Drawing for the job (mm, zero at the part's lowest x, y, z). Round coordinates to 2 decimals unless told otherwise and drop trailing zeros. Write each loop counter-clockwise with the first axis right and the second up, starting at its lowest first coordinate (ties: lowest second). Pieces come first, ordered by that corner, then holes. Notation, with made-up numbers: (21.25, 56.5) - (41.25, 56.5) arc R26 cw to (41.25, 77.5) - close; hole circle Ø7 at (87, 31). An arc over 180 degrees is marked (long way). One line per question, with ' | ' between items.
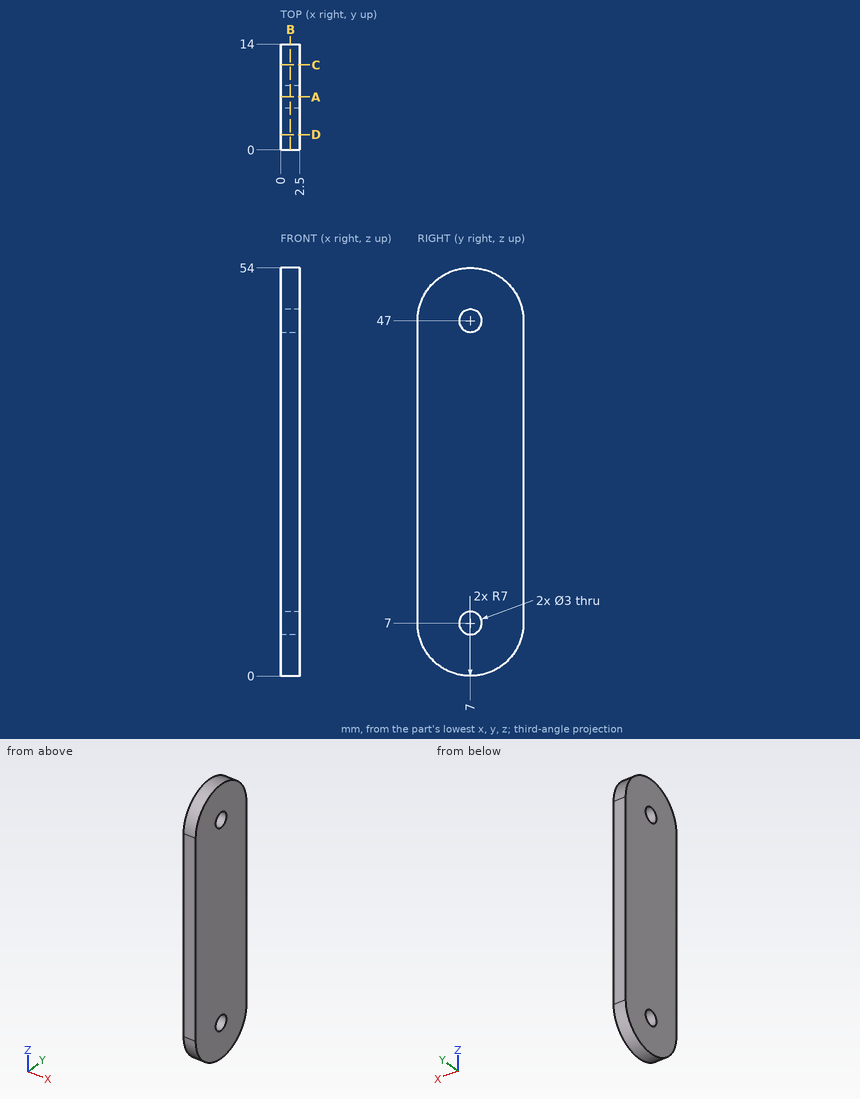
Q1. Saw through at B-B, the plane x = 1.3. List the corners of the cut face in (y, z), then the cut area to 3 significant figures.
Found:
outline: (0, 7) arc R7 ccw to (14, 7) - (14, 47) arc R7 ccw to (0, 47) - close; hole circle Ø3 at (7, 7); hole circle Ø3 at (7, 47) | area: 700 mm^2
Q2. Saw through at A-A, the plane y = 7. List the corners of the cut face in (x, z), then the cut area to 3 significant figures.
Found:
outline: (0, 0) - (2.5, 0) - (2.5, 5.5) - (0, 5.5) - close; (0, 8.5) - (2.5, 8.5) - (2.5, 45.5) - (0, 45.5) - close; (0, 48.5) - (2.5, 48.5) - (2.5, 54) - (0, 54) - close | area: 120 mm^2
Q3. Drill centre lines: L1, parallel to Y at x = 0.75, z = 7; L2, parallel to Z at x = 1.5, y = 7.5; L3, parallel to Z at x = 2.4, y = 6.75. Where is each one in solid material? Low to high. Write a range as from..to.
Found:
L1: 0..5.5, 8.5..14 | L2: 0.02..5.59, 8.41..45.59, 48.41..53.98 | L3: 0..5.52, 8.48..45.52, 48.48..54
Q4. Saw through at D-D, the plane y = 2. List the corners of the cut face in (x, z).
Found:
outline: (0, 2.1) - (2.5, 2.1) - (2.5, 51.9) - (0, 51.9) - close
Q5. Saw through at C-C, the plane y = 11.25. List the corners of the cut face in (x, z), then the cut area to 3 significant figures.
Found:
outline: (0, 1.44) - (2.5, 1.44) - (2.5, 52.56) - (0, 52.56) - close | area: 128 mm^2
Q6. Drop a flat-ended pin along its axis: pin 1 (1 mm diameter, centred on x = 0.5, y = 8.5, fed in from +Z). Give the stop position or say it passes through.
Found:
pin 1: z = 53.93
